Autodesk Inventor part; units mm, degrees
ref_plane "YZ Plane" through (0, 0, 0) normal (1, 0, 0) x (0, 1, 0)
ref_plane "XZ Plane" through (0, 0, 0) normal (0, 1, 0) x (-1, 0, 0)
ref_plane "XY Plane" through (0, 0, 0) normal (0, 0, 1) x (1, 0, 0)
sketch "スケッチ2" plane through (0, 0, 0) normal (0, 1, 0) x (-1, 0, 0)
  arc A0 (186.0286, -63.1802) -> (352.6649, -47.4935) centre (165.9229, 1043.3137) ccw
  arc A1 (138.8299, -62.6406) -> (186.0286, -63.1802) centre (171.5405, 734.1521) ccw
  arc A2 (52.1426, -47.2314) -> (138.8299, -62.6406) centre (152.2575, 264.4411) ccw
  arc A3 (2.1008, -22.6524) -> (52.1426, -47.2314) centre (110.8425, 135.5101) ccw
  arc A4 (-12.1054, -8.8578) -> (2.1008, -22.6524) centre (35.5695, 26.0271) ccw
  arc A5 (-4.5779, 14.2844) -> (-12.1054, -8.8578) centre (0, 0) ccw
  arc A6 (16.7232, 17.0724) -> (-4.5779, 14.2844) centre (13.7336, -42.8531) ccw
  arc A7 (94.7165, 2.6851) -> (16.7232, 17.0724) centre (1.7751, -282.555) ccw
  arc A8 (94.7165, 2.6851) -> (99.4705, 1.147) centre (466.4821, 1143.6454) ccw
  arc A9 (99.4705, 1.147) -> (352.0248, -39.551) centre (359.437, 810.4167) ccw
  arc A10 (352.6649, -47.4935) -> (352.0248, -39.551) centre (351.99, -43.5508) ccw
  circle A11 centre (33.0346, -3.4541) radius 6
  circle A12 centre (243.4846, -47.452) radius 6
  point P0 (0, 0)
extrude "押し出し2" add sketch "スケッチ2" along normal mid plane 186
ref_plane "作業平面1" through (-49.9941, -10.2, 38.589) normal (-0.2588, 0, 0.9659) x (0.9659, 0, 0.2588)
sketch "スケッチ3" plane through (-49.9941, -10.2, 38.589) normal (-0.2588, 0, 0.9659) x (0.9659, 0, 0.2588)
  line L0 (18, 13.4) -> (18, 7)
  line L1 (0, -2.3) -> (11, -2.3)
  line L2 (-7, 7) -> (-7, 13.4)
  line L3 (11, 22.7) -> (0, 22.7)
  line L4 (18, -2.3) -> (-7, -2.3)
  line L5 (-7, -2.3) -> (-7, 22.7)
  line L6 (-7, 22.7) -> (18, 22.7)
  line L7 (18, 22.7) -> (18, -2.3)
  line L8 (-8, -3.3) -> (19, -3.3)
  line L9 (19, -3.3) -> (19, 23.7)
  line L10 (19, 23.7) -> (-8, 23.7)
  line L11 (-8, 23.7) -> (-8, -3.3)
  point P0 (38.303, 10.2)
  dimension "d6" = 1
extrude "押し出し3" cut sketch "スケッチ3" against normal blind 60 contours L0 L7 L4 L1 L5 L2 L6 L3 | L11 L10 L9 L8
properties part number "mainflap for center"
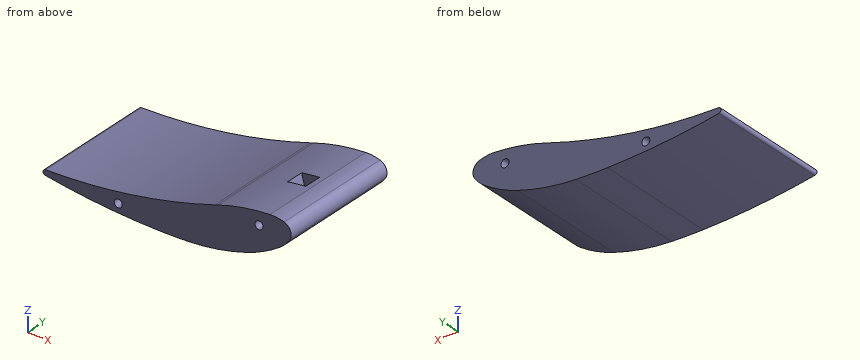
The model under review builds one solid part; all positions refer to its coordinate system, in mm. Give positions to 0.01 mm unless a question says otherwise; leave off trailing zeros. Write each loop counter-clockwise with the first axis right and the second up, starting at its lowest first coordinate (ties: lowest second). Pieces come first, ordered by that corner, then holes. Notation, with made-up numbers: (78.25, 39) -> (119.25, 39) arc R21 cw to (119.25, 71) -> close; hole circle Ø1 at (-14, 83.25). An arc over 180 degrees is marked (long way). Put each result on its own line as item: value.
(1) We need section D-D, the plane x = -291.5. Give the boundary of the cut face in (y, z) (3 decimals).
Results are:
outline: (-93, -56.215) -> (93, -56.215) -> (93, -36.864) -> (-93, -36.864) -> close
(2) For pin 1 Ø2 at (y, z) = (24, -44.5) entering from -X; pin 2 Ø1.5 at (y, z) = (24, -35) entering from +X; pin 3 Ø1.5 at (y, z) = (-53.5, -23) entering from +X, all flat-tipped, find the tip position at first contact; note any pin that passes through.
Results are:
pin 1: x = -355.99
pin 2: x = -21.28
pin 3: x = -1.52
(3) We need section C-C, the plane z = 7. Give the boundary of the cut face in (x, y), and give its area (3 significant figures).
Results are:
outline: (-80.25, -93) -> (13.27, -93) -> (13.27, 93) -> (-80.25, 93) -> close; hole (-49.81, -13.5) -> (-21.86, -13.5) -> (-21.86, 13.5) -> (-49.81, 13.5) -> close
area: 16,600 mm²
(4) To check wall thickness, follow probe 1 along Y at (x, z) = (-43, -2); probe 2 along Z at (x, y) = (-254.5, -4.5); probe 3 along Z at (x, y) = (-11.5, 2.5). State the ranges of each line that lie inside material, in increasing order. Write a range as from..to.
Results are:
probe 1: -93..-13.5, 13.5..93
probe 2: -59.81..-33.08
probe 3: -28.72..17.11
(5) We need section B-B, the plane y = 4.5. Give the boundary of the cut face in (x, z).
Results are:
outline: (-352.66, -47.49) arc R1106.67 ccw to (-186.03, -63.18) arc R797.54 ccw to (-138.83, -62.64) arc R327.36 ccw to (-52.14, -47.23) arc R191.94 ccw to (-2.1, -22.65) arc R59.07 ccw to (12.11, -8.86) arc R15 ccw to (4.58, 14.28) arc R60 ccw to (-16.72, 17.07) arc R300 ccw to (-24.43, 16.59) -> (-16.11, -14.45) -> (-42.19, -21.44) -> (-51.5, 13.3) arc R300 ccw to (-94.72, 2.69) arc R1203.96 cw to (-99.47, 1.15) arc R850 cw to (-352.02, -39.55) arc R4 ccw to start; hole circle Ø12 at (-243.48, -47.45)
(6) We need section A-A, the plane y = -47. Give the boundary of the cut face in (x, z), and give its area (3 significant figures).
Results are:
outline: (-352.66, -47.49) arc R1106.67 ccw to (-186.03, -63.18) arc R797.54 ccw to (-138.83, -62.64) arc R327.36 ccw to (-52.14, -47.23) arc R191.94 ccw to (-2.1, -22.65) arc R59.07 ccw to (12.11, -8.86) arc R15 ccw to (4.58, 14.28) arc R60 ccw to (-16.72, 17.07) arc R300 ccw to (-94.72, 2.69) arc R1203.96 cw to (-99.47, 1.15) arc R850 cw to (-352.02, -39.55) arc R4 ccw to start; hole circle Ø12 at (-243.48, -47.45); hole circle Ø12 at (-33.03, -3.45)
area: 14,200 mm²
